Design review of the part shown in the three views and the two pictorial views. Dimensions are in mm from the part's minimum x, y and z. A direction names the side the tool comes from. Give positions to 0.01 mm unless a question says otherwise; leave off trailing zeros. Order: outer loops, then holes, each group sorted by start corner. A loop starts at its lowest first (then second) coordinate and runs counter-clockwise, first axis right, second up.
Item 1: Machinability: for the marked faces 4, 5 and 6, which of the approach directions +Z, -Z, +X, -X, +Y, -Y give a long, thin tool a straight path to every point of the face, cutting with its end or side? Answer none if there is none.
Item 2: Consider section D-D (z = 35). Give the boundary of the cut face in (x, y), plus the area to 3 significant figures.
Item 3: For probe 1 along Y at (x, z) = (28.65, 35); probe 2 along Z at (x, y) = (19, 25), list the stretches that pass through material, from the lowest coordinate up.
Item 4: Consider section B-B (x = 15). Give the boundary of the cut face in (y, z), plus the area to 4 significant figures.
Item 5: Consider section A-A (y = 15). Give the boundary of the cut face in (x, z), plus the area to 4 significant figures.
Item 6: Consider section C-C (y = 2). Give the boundary of the cut face in (x, z).
Item 7: For P1, Ø12, axis at x = 27, y = 13.5, coming from the -Z side; P2, Ø5, axis at x = 4, y = 9, coming from the +Z side; P3, Ø2.5, axis at y = 16.5, z = 11.5, coming from the -X side; P4, Ø2, axis at x = 10.5, z = 43, coming from the +Y side, all flat-tipped, find the tip position at first contact; note any pin that passes through.
Item 8: The part is to be moulded in two halves that separate along Z. For the marked faces 1, 2 and 3, say which applies: released by +Z, released by -Z, zero draft, split by the parting line, or undercut.
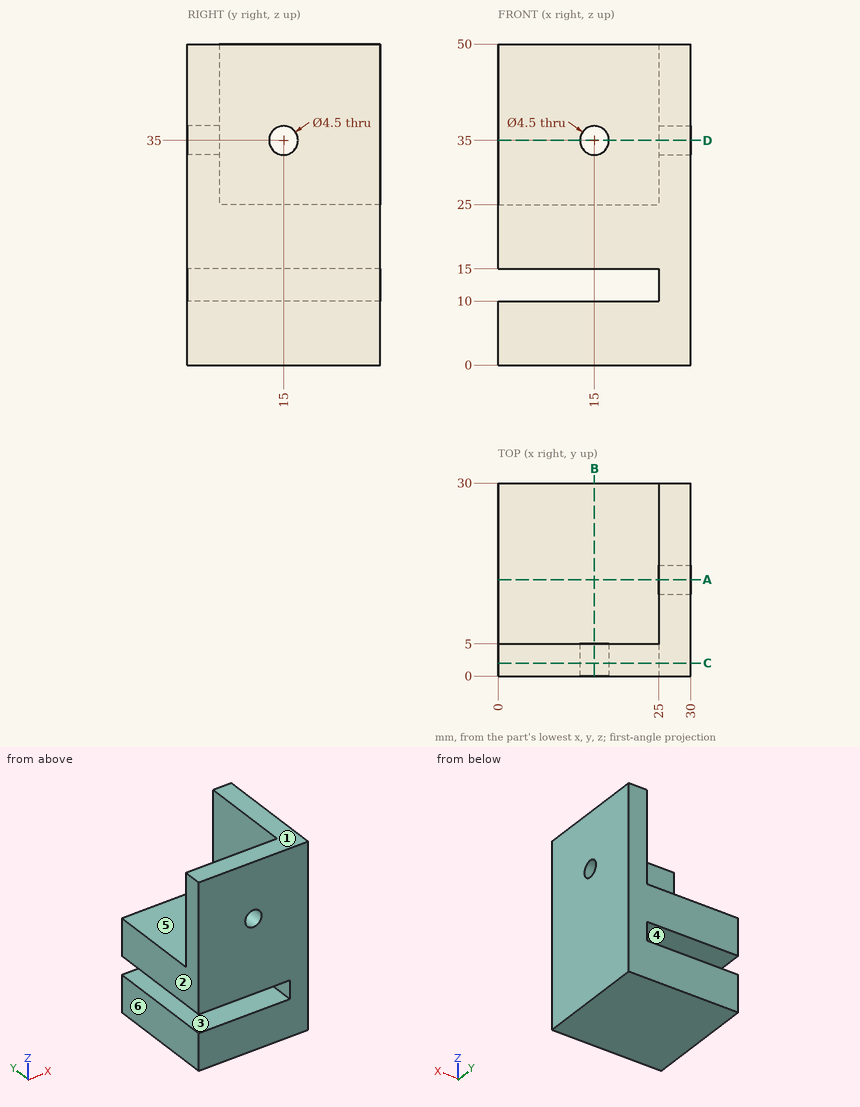
Resolved:
1. face 4: -X, +Y, -Y
1. face 5: +Z, -X, +Y
1. face 6: +Z, -Z, -X, +Y, -Y
2. outline: (0, 0) - (12.75, 0) - (12.75, 5) - (0, 5) - close; (17.25, 0) - (30, 0) - (30, 12.75) - (25, 12.75) - (25, 5) - (17.25, 5) - close; (25, 17.25) - (30, 17.25) - (30, 30) - (25, 30) - close
2. area: 230 mm2
3. probe 1: y = 0 to 12.75, 17.25 to 30
3. probe 2: z = 0 to 10, 15 to 25
4. outline: (0, 0) - (30, 0) - (30, 10) - (0, 10) - close; (0, 15) - (30, 15) - (30, 25) - (5, 25) - (5, 32.75) - (0, 32.75) - close; (0, 37.25) - (5, 37.25) - (5, 50) - (0, 50) - close
4. area: 702.5 mm2
5. outline: (0, 0) - (30, 0) - (30, 32.75) - (25, 32.75) - (25, 25) - (0, 25) - (0, 15) - (25, 15) - (25, 10) - (0, 10) - close; (25, 37.25) - (30, 37.25) - (30, 50) - (25, 50) - close
5. area: 727.5 mm2
6. outline: (0, 0) - (30, 0) - (30, 50) - (0, 50) - (0, 15) - (25, 15) - (25, 10) - (0, 10) - close; hole circle Ø4.5 at (15, 35)
7. P1: stops at z = 0
7. P2: stops at z = 25
7. P3: stops at x = 25
7. P4: stops at y = 5
8. face 1: released by +Z
8. face 2: zero draft
8. face 3: undercut
